Here's how the part is built. I have some questions about the finished solid (model axes, mm). A direction names the side the tool comes from. Coordinates: 2 decimals unless noted, no trailing zeros.
Item 1: I want a section at A-A (z = 6.75). Count the separate pieces of the cut face and the enclosed holes in it, and give its area (3 significant figures).
Item 2: Please list where these lines run through material, in increasing order: line 1 (Y direction, x = -12, z = 6.5); line 2 (Z direction, x = -12, y = -6.25).
Item 3: If we mould it in two halves opening along Y, with no side actions, what happens to faces 1 (the face through (16, 0, 5)), 2 (the face through (20.085, 0, 5))? For each: pulls with the +Y half, pulls with the -Y half, needs draft (parallel to the pull), parting line crosses it, or undercut.
Item 4: For faces 3 (the face through (-3.072, 0, 8)), 4 (the face through (-19.926, 0, 5)), which set-ups out of +Z, -Z, +X, -X, +Y, -Y let a thin tool reach every point of the face, with its end or its side?
from build123d import *

# Parameters (mm, degrees)
SKETCH_W            = 40.010176
SKETCH_H            = 19.766459
PAD_DEPTH           = 10
SKETCH001_W         = 0.949318
SKETCH001_H         = 16.960248
POCKET_DEPTH        = 5
LINEARPATTERN_COUNT = 8
LINEARPATTERN_PITCH = 4.714286


with BuildPart() as part:
    # Sketch → Pad (new body)
    with BuildSketch(Plane.XY):
        with Locations((0.079543, 0.039771)):
            Rectangle(SKETCH_W, SKETCH_H)
    extrude(amount=PAD_DEPTH)

    # Sketch001 (on Face6 of Pad) → Pocket (cut)
    with BuildSketch(Plane.XY.offset(10)):
        with Locations((-16.740425, 0)):
            Rectangle(SKETCH001_W, SKETCH001_H)
    pocket = extrude(amount=-POCKET_DEPTH, mode=Mode.SUBTRACT)

    # LinearPattern: Pocket ×8
    with Locations(*[(i * LINEARPATTERN_PITCH, 0, 0) for i in range(1, LINEARPATTERN_COUNT)]):
        add(pocket, mode=Mode.SUBTRACT)


solid = part.part
Answer:
1. separate pieces: 1
1. enclosed holes: 8
1. area: 662 mm2
2. line 1: y = -9.84 to -8.48, 8.48 to 9.92
2. line 2: z = 0 to 5
3. face 1: undercut
3. face 2: needs draft
4. face 3: +Z
4. face 4: +Z, -Z, -X, +Y, -Y
